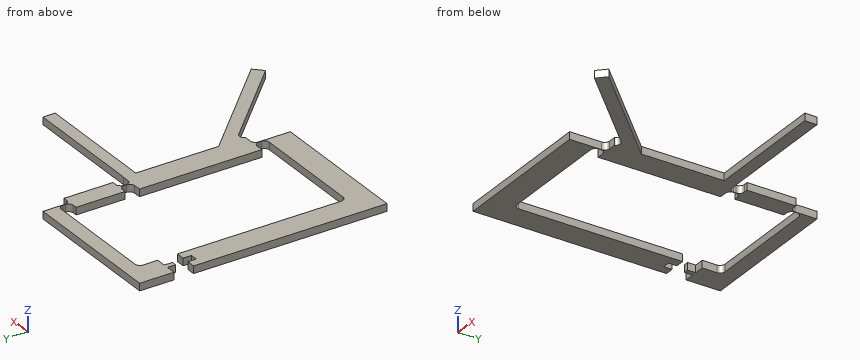
```python
from build123d import *

# Parameters (mm, degrees)
BOSS_EXTRUDE1_DEPTH = 3
FILLET1_R           = 2


with BuildPart() as part:
    # Sketch2 → Boss-Extrude1 (new body)
    with BuildSketch(Plane.XY):
        Polygon((0, 0), (0, 79), (3.5, 79), (3.5, 75.566666667), (6.5, 75.566666667), (6.5, 79), (10, 79), (10, 10), (59.8, 10), (59.8, 15), (54.9, 15), (54.9, 65), (59.8, 65), (59.8, 70), (56.15, 70), (56.15, 90), (59.8, 90), (59.8, 95), (10, 95), (10, 87), (6, 87), (6, 83.666666667), (4, 83.666666667), (4, 87), (0, 87), (0, 91), (0, 101), (60, 101), (60, 95), (60, 90), (63.65, 90), (63.65, 70), (60, 70), (60, 65), (64.9, 65), (64.9, 64.9), (114.9, 64.9), (114.9, 59.9), (64.9, 59.9), (64.9, 26.071055471), (103.790928501, -12.819737276), (100.255400766, -16.355277353), (64.9, 19), (64.9, 15), (60, 15), (60, 10), (60, 0), align=None)
    extrude(amount=BOSS_EXTRUDE1_DEPTH)

    # Fillet1
    # the kernel refuses this fillet: 2 mm, written as the material it adds along each edge
    with BuildSketch(Plane(origin=(59.8, 15, 0), x_dir=(-1, 0, 0), z_dir=(0, 0, 1)), Plane(origin=(60, 15, 0), x_dir=(0, -1, 0), z_dir=(0, 0, 1)), Plane(origin=(60, 70, 0), x_dir=(0, -1, 0), z_dir=(0, 0, 1)), Plane(origin=(60, 65, 0), x_dir=(1, 0, 0), z_dir=(0, 0, 1)), Plane(origin=(59.8, 65, 0), x_dir=(0, 1, 0), z_dir=(0, 0, 1)), Plane(origin=(59.8, 70, 0), x_dir=(-1, 0, 0), z_dir=(0, 0, 1)), Plane(origin=(59.8, 95, 0), x_dir=(-1, 0, 0), z_dir=(0, 0, 1)), Plane(origin=(60, 90, 0), x_dir=(1, 0, 0), z_dir=(0, 0, 1)), Plane(origin=(59.8, 90, 0), x_dir=(0, 1, 0), z_dir=(0, 0, 1)), Plane(origin=(10, 10, 0), x_dir=(1, 0, 0), z_dir=(0, 0, 1)), Plane(origin=(10, 95, 0), x_dir=(0, -1, 0), z_dir=(0, 0, 1)), Plane(origin=(59.8, 10, 0), x_dir=(0, 1, 0), z_dir=(0, 0, 1))) as fillet1_piece_1:
        with BuildLine():
            CenterArc((FILLET1_R, FILLET1_R), FILLET1_R, 180, 90)
            Line((0, FILLET1_R), (-FILLET1_R * 0.02, FILLET1_R))
            Line((-FILLET1_R * 0.02, FILLET1_R), (-FILLET1_R * 0.02, -FILLET1_R * 0.02))
            Line((-FILLET1_R * 0.02, -FILLET1_R * 0.02), (FILLET1_R, -FILLET1_R * 0.02))
            Line((FILLET1_R, -FILLET1_R * 0.02), (FILLET1_R, 0))
        make_face()
    extrude(amount=3)
    with BuildSketch(Plane(origin=(64.9, 19, 0), x_dir=(0, -1, 0), z_dir=(0, 0, 1))) as fillet1_piece_2:
        with BuildLine():
            CenterArc((4.70139372, 1.87297807), FILLET1_R, 135.0001, 114.469955898)
            Line((3.287177689, 3.287189164), (3.258893369, 3.315473386))
            Line((3.258893369, 3.315473386), (-0.028284321, 0.028284222))
            Line((-0.028284321, 0.028284222), (0, -0.04))
            ThreePointArc((0, -0.04), (2, -0.04), (3.985972126, -0.037459561))
            Line((3.985972126, -0.037459561), (4, 0))
        make_face()
    extrude(amount=3)


solid = part.part
```
Input: part model. Units: mm. Frame: model coordinates. Give positions to 0.01 mm unless a question says otherwise; leave off trailing zeros. Order: outer loops, then holes, each group sorted by start corner. A loop starts at its lowest first (then second) coordinate and runs counter-clockwise, first axis right, second up. Notation, with made-up numbers: M 87.5,18.25 L 101.5,18.25 A25 ccw 101.5,31.25 Z; hole C -29,-12.5 d5. An arc over 180 degrees is marked long. One line per question, with ' | ' between items. Start each with the question number.
1. Material intervals for probe 1 along Y at (x, z) = (55, 1.1); probe 2 along X at (y, z) = (50.5, 0.5); probe 3 along Y at (x, z) = (26.5, 1.65), sorted ascending. Write a range as [from, to].
2. Section query A-A (y = 85). Return the cut outline in (x, z), and give its area (3 significant figures).
3. First-contact query: pin 1 Ø0.9 at (x, z) = (25, 1) entering from -Y; pin 2 Ø1 at (x, z) = (81.5, 2) entering from -Y; pin 3 Ø1.1 at (y, z) = (67.5, 1) entering from -X; pin 4 Ø0.9 at (y, z) = (80, 1.5) entering from +X. Flat tips, straight axial feed; report the tip coordinate or a pass-through.
4. Section query B-B (x = 8). Return the cut outline in (y, z).
Here are the results:
1) probe 1: [0, 10], [15, 65], [95, 101] | probe 2: [0, 10], [54.9, 64.9] | probe 3: [0, 10], [95, 101]
2) outline: M 4,0 L 6,0 L 6,3 L 4,3 Z; M 56.15,0 L 63.65,0 L 63.65,3 L 56.15,3 Z | area: 28.5 mm²
3) pin 1: y = 0 | pin 2: y = 1.9 | pin 3: x = 0 | pin 4: x = 63.65
4) outline: M 0,0 L 79,0 L 79,3 L 0,3 Z; M 87,0 L 101,0 L 101,3 L 87,3 Z
